```python
from build123d import *

# Parameters (mm, degrees)
EXTRUDE_1_DEPTH = 10
FILLET_1_R      = 2
FILLET_2_R      = 1


# Some blends are built 0.0001 mm under size
with BuildPart() as part:
    # Эскиз1 → Бобышка-Вытянуть1 (new body)
    with BuildSketch(Plane.XY):
        with BuildLine():
            ThreePointArc((3.872983346, -1), (0, 4), (-3.872983346, -1))
            Line((-3.872983346, -1), (-7, -1))
            Line((-7, -1), (-7, 7))
            Line((-7, 7), (7, 7))
            Line((7, 7), (7, -1))
            Line((7, -1), (3.872983346, -1))
        make_face()
        Polygon((7, 0.025778788), (59.392231378, -3.446827136), (60.607768622, 3.446827136), (7, 7), align=None)
        Polygon((59.392231378, -3.446827136), (92.245234414, -14.802793492), (92.245234414, -12.85), (107.754765586, -12.85), (60.607768622, 3.446827136), align=None)
        Polygon((104.55, -14.85), (104.55, -20.85), (107.754765586, -20.85), (107.754765586, -12.85), (92.245234414, -12.85), (92.245234414, -20.85), (95.45, -20.85), (95.45, -14.85), align=None)
    extrude(amount=EXTRUDE_1_DEPTH)

    # Скругление1
    # the kernel refuses this fillet: 2 mm, written as the material it adds along each edge
    with BuildSketch(Plane(origin=(59.392231378, -3.446827136, 0), x_dir=(0.9451302843245073, -0.32669365719688503, 0), z_dir=(0, 0, 1))) as fillet_1_piece_1:
        with BuildLine():
            CenterArc((FILLET_1_R * 0.134104869986, -FILLET_1_R), FILLET_1_R, 90, 15.276145222)
            Line((-FILLET_1_R * 0.129366569023, -FILLET_1_R * 0.0353328030732), (0, 0))
            Line((0, 0), (FILLET_1_R * 0.134104869986, 0))
        make_face()
    extrude(amount=10)
    with BuildSketch(Plane(origin=(7, 0.025778788, 0), x_dir=(0, -1, 0), z_dir=(0, 0, 1))) as fillet_1_piece_2:
        with BuildLine():
            CenterArc((2.115543143, 1.677025238), FILLET_1_R, 176.207928907, 60.775458648)
            Line((0.119921883, 1.809296875), (0, 0))
            Line((0, 0), (1.025778788, 0))
        make_face()
    extrude(amount=10)
    with BuildSketch(Plane(origin=(92.245234414, -14.802793492, 0), x_dir=(-0.945130284324508, 0.3266936571968835, 0), z_dir=(0, 0, 1))) as fillet_1_piece_3:
        with BuildLine():
            CenterArc((FILLET_1_R * 0.712395268642, FILLET_1_R), FILLET_1_R, 199.068216315, 70.931783685)
            Line((-FILLET_1_R * 0.232735015682, FILLET_1_R * 0.673306342803), (0, 0))
            Line((0, 0), (FILLET_1_R * 0.712395268642, 0))
        make_face()
    extrude(amount=10)
    # the kernel refuses this fillet: 2 mm, written as the material it takes off along each edge
    with BuildSketch(Plane(origin=(-7, -1, -5), x_dir=(1, 0, 0), z_dir=(0, 0, 1)), Plane(origin=(-7, 7, -5), x_dir=(0, -1, 0), z_dir=(0, 0, 1)), Plane(origin=(107.754765586, -20.85, -5), x_dir=(0, 1, 0), z_dir=(0, 0, 1)), Plane(origin=(92.245234414, -20.85, -5), x_dir=(1, 0, 0), z_dir=(0, 0, 1))) as fillet_1_2_piece_1:
        with BuildLine():
            CenterArc((FILLET_1_R, FILLET_1_R), FILLET_1_R, 180, 90)
            Line((0, FILLET_1_R), (0, 0))
            Line((0, 0), (FILLET_1_R, 0))
        make_face()
    extrude(amount=20, mode=Mode.SUBTRACT)
    with BuildSketch(Plane(origin=(107.754765586, -12.85, -3.561976343), x_dir=(-0.9451302843245086, 0.3266936571968812, 0), z_dir=(0, 0, 1))) as fillet_1_2_piece_2:
        with BuildLine():
            CenterArc((FILLET_1_R * 0.712395268642, FILLET_1_R), FILLET_1_R, 199.068216315, 70.931783685)
            Line((-FILLET_1_R * 0.232735015682, FILLET_1_R * 0.673306342803), (0, 0))
            Line((0, 0), (FILLET_1_R * 0.712395268642, 0))
        make_face()
    extrude(amount=17.123952686, mode=Mode.SUBTRACT)
    with BuildSketch(Plane(origin=(7, 7, -0.165520739), x_dir=(-1, 0, 0), z_dir=(0, 0, 1))) as fillet_1_2_piece_3:
        with BuildLine():
            CenterArc((FILLET_1_R * 0.0331041478527, FILLET_1_R), FILLET_1_R, 266.207928907, 3.792071093)
            Line((-FILLET_1_R * 0.0330316706273, FILLET_1_R * 0.00218936991332), (0, 0))
            Line((0, 0), (FILLET_1_R * 0.0331041478527, 0))
        make_face()
    extrude(amount=10.331041479, mode=Mode.SUBTRACT)
    with BuildSketch(Plane(origin=(60.607768622, 3.446827136, -0.67052435), x_dir=(-0.9978106300866822, 0.06613581847999181, 0), z_dir=(0, 0, 1))) as fillet_1_2_piece_4:
        with BuildLine():
            CenterArc((FILLET_1_R * 0.134104869986, FILLET_1_R), FILLET_1_R, 254.723854778, 15.276145222)
            Line((-FILLET_1_R * 0.129366569023, FILLET_1_R * 0.0353328030732), (0, 0))
            Line((0, 0), (FILLET_1_R * 0.134104869986, 0))
        make_face()
    extrude(amount=11.3410487, mode=Mode.SUBTRACT)

    # Скругление2
    fillet_2_edges = [part.edges().sort_by_distance(p)[0] for p in [
        (7, -1, 5),
        (3.872983346, -1, 5),
        (-3.872983346, -1, 5),
    ]]
    fillet(fillet_2_edges, radius=FILLET_2_R - 0.0001)  # a hair under: the kernel refuses the full size


solid = part.part
```
Could you check a few things on this model? Use its own coordinates, in mm. A direction names the side the tool comes from. Give positions to 0.01 mm unless a question says otherwise; leave off trailing zeros. Loops run counter-clockwise (first coordinate to the right, second up) from the corner with the lowest first, then second, coordinate; pieces in that order, holes last. Notation, with made-up numbers: (47, 77) - (64, 77) arc R29 ccw to (64, 99) - close; hole circle Ø9 at (-29.75, 54). An arc over 180 degrees is marked (long way). Answer in a Markdown table with one row per item. Add a question column.
Q1. For pin 1 (0.8 mm diameter, centred on y = -18, z = 4, fed in from -X); pin 2 (1.7 mm diameter, centred on x = 6, z = 4, fed in from -Y); pin 3 (2 mm diameter, centred on y = -1.5, z = 5.5, fed in from -X), each with a flat end and sliding along its axis, tell me the tip position at first contact or that it passes through.
Q2. Please list where these lines run through material, in increasing order: L1, parallel to X at y = -15, z = 9.25; L2, parallel to Y at x = 0, z = 9; L3, parallel to Y at x = 69, z = 5.75. Write a range as from..to.
Q3. Which directions (+Z, -Z, +X, -X, +Y, -Y) give clear straight access to the entire face, cutting with the end or side of a thin tool? Please do faces 1 (the face through (95.45, -18, 5)), 2 (the face through (1, 7, 5)), 3 (the face through (92.245, -18, 5)).
Q4. If we section it at C-C (y = -8): List the corners of the cut face in (x, z) for me.
Q5. We'd pull the mould along X, two halves only. Please class faces 4 (the face through (33.615, -1.738, 4.93)), 5 (the face through (83.95, -4.62, 4.93)), 6 (the face through (-6.4, 6.43, 4.93)): +X half, -X half, draft (parallel to the pull), parting line (faces both ways), or undercut.
Q6. If we section it at B-B (x = 0): List the corners of the cut face in (y, z) for me, plus the area to 3 significant figures.
The answers:
| question | item | result |
|---|---|---|
| 1 | pin 1 | stops at x = 92.25 |
| 1 | pin 2 | stops at y = -1 |
| 1 | pin 3 | stops at x = -6.32 |
| 2 | L1 | x = 91.82..95.45, 104.55..107.75 |
| 2 | L2 | y = 4..7 |
| 2 | L3 | y = -6.77..0.55 |
| 3 | face 1 | +Z, -Z, -Y |
| 3 | face 2 | +Z, -Z, +X, -X, +Y |
| 3 | face 3 | +Z, -Z, -X, -Y |
| 4 | outline | (72.56, 0) - (93.72, 0) - (93.72, 10) - (72.56, 10) - close |
| 5 | face 4 | undercut |
| 5 | face 5 | +X half |
| 5 | face 6 | -X half |
| 6 | outline | (4, 0) - (7, 0) - (7, 10) - (4, 10) - close |
| 6 | area | 30.0 mm^2 |
